For this review, take the finished solid that the model builds, in its own axes (mm). A direction names the side the tool comes from. Round coordinates to 2 decimals unless told otherwise and drop trailing zeros. Write each loop counter-clockwise with the first axis right and the second up, starting at its lowest first coordinate (ties: lowest second). Pieces come first, ordered by that corner, then holes.
from build123d import *

# Parameters (mm, degrees)
F0_W     = 41.342575
F0_H     = 85.221954
F1_DEPTH = 34.889519
F2_W     = 41.342575
F2_H     = 76.076616
F3_DEPTH = 33.270478
F4_W     = 7.088874
F4_H     = 7.146471
F5_DEPTH = 34.3295
F6_W     = 7.894669
F6_H     = 6.943033
F7_DEPTH = 34.407657


with BuildPart() as f1:
    # F0 (on Top) → F1 (new body)
    with BuildSketch(Plane.XY):
        with Locations((20.671287, 0.345733)):
            Rectangle(F0_W, F0_H)
    extrude(amount=F1_DEPTH)

    # F2 (on face) → F3 (join)
    with BuildSketch(Plane.XY.offset(34.889519)):
        with Locations((20.671287, -37.692575)):
            Rectangle(F2_W, F2_H)
    extrude(amount=F3_DEPTH)

    # F4 (on face) → F5 (join)
    with BuildSketch(Plane(origin=(0, 0, 34.889519), x_dir=(1, 0, 0), z_dir=(0, 0, -1))):
        with Locations((3.544437, 72.157647)):
            Rectangle(F4_W, F4_H)
    extrude(amount=F5_DEPTH)

    # F6 (on face) → F7 (join)
    with BuildSketch(Plane(origin=(0, 0, 34.889519), x_dir=(1, 0, 0), z_dir=(0, 0, -1))):
        with Locations((37.39524, 72.259366)):
            Rectangle(F6_W, F6_H)
    extrude(amount=F7_DEPTH)


solid = f1.part
(1) For pin 1 Ø2 at (x, y) = (5, -71.5) entering from -Z; pin 2 Ø6 at (x, z) = (36, 42) entering from +Y; pin 3 Ø3.5 at (x, y) = (36.5, -72) entering from -Z; pin 4 Ø7.5 at (y, z) = (-71, 22) entering from -X, all flat-tipped, find the tip position at first contact; note any pin that passes through.
Geometry check:
pin 1: stops at z = 0.56
pin 2: stops at y = 0.35
pin 3: stops at z = 0.48
pin 4: stops at x = 0
(2) We need section D-D, the plane y = 16. Give the boundary of the cut face in (x, z), and give its area (3 significant figures).
Geometry check:
outline: (0, 0) - (41.34, 0) - (41.34, 34.89) - (0, 34.89) - close
area: 1,440 mm2
(3) For line 1 along Y through (x, z) = (37.5, 25); line 2 along Y through (x, z) = (3.5, 20); line 3 along Y through (x, z) = (24, 43), list the stretches that pass through material, from the lowest coordinate up.
Geometry check:
line 1: y = -75.73 to -68.79, -42.27 to 42.96
line 2: y = -75.73 to -68.58, -42.27 to 42.96
line 3: y = -75.73 to 0.35
(4) We need section B-B, the plane x = 4.5. Give the boundary of the cut face in (y, z), and give its area (3 significant figures).
Geometry check:
outline: (-75.73, 0.56) - (-68.58, 0.56) - (-68.58, 34.89) - (-42.27, 34.89) - (-42.27, 0) - (42.96, 0) - (42.96, 34.89) - (0.35, 34.89) - (0.35, 68.16) - (-75.73, 68.16) - close
area: 5,750 mm2
(5) Mouldability with a two-part tool opening along X and no side actions: class faces 1 (the face through (33.448, -72, 18)), 2 (the face through (3, -72, 0.56)), 3 (the face through (0, -72, 18)) as pulls with the +X half, pulls with the -X half, needs draft (parallel to the pull), parting line crosses it, or undercut.
Geometry check:
face 1: undercut
face 2: needs draft
face 3: pulls with the -X half
(6) We need section C-C, the plane x = 13. Give the boundary of the cut face in (y, z).
Geometry check:
outline: (-75.73, 34.89) - (-42.27, 34.89) - (-42.27, 0) - (42.96, 0) - (42.96, 34.89) - (0.35, 34.89) - (0.35, 68.16) - (-75.73, 68.16) - close
(7) For faces 4 (the face through (37, -68.788, 18)), 5 (the face through (7.089, -72, 18)), 6 (the face through (20, -42.265, 17)), 7 (the face through (37, -72, 0.482)), list the 3-axis set-ups (+Z, -Z, +X, -X, +Y, -Y) from which the entire face can be reached by the end or side of a thin tool; tool diameter is ignored.
Geometry check:
face 4: -Z, +X
face 5: -Z, -Y
face 6: -Z, +X, -X
face 7: -Z, +X, -X, -Y
(8) We need section A-A, the plane z = 27.5. Give the boundary of the cut face in (x, y).
Geometry check:
outline: (0, -75.73) - (7.09, -75.73) - (7.09, -68.58) - (0, -68.58) - close; (0, -42.27) - (41.34, -42.27) - (41.34, 42.96) - (0, 42.96) - close; (33.45, -75.73) - (41.34, -75.73) - (41.34, -68.79) - (33.45, -68.79) - close
